Read the model definition and answer for the solid it produces. Units are mm, in the model's axes. Face numbers are marked on the shaded views. A direction names the side the tool comes from. Round coordinates to 2 decimals unless told otherwise and drop trailing zeros. Write each loop counter-clockwise with the first axis right and the second up, starting at its lowest first coordinate (ties: lowest second). Pieces come first, ordered by that corner, then holes. Notation, with made-up numbers: (-20, -9) -> (-3, -9) arc R6 cw to (-3, 1) -> close; hole circle Ø2 at (13, 86). An arc over 180 degrees is marked (long way). Return JSON: item names as keys, results as strings.
from build123d import *

# Parameters (mm, degrees)
SKETCH1_R                  = 1.75
BOSS_EXTRUDE1_DEPTH        = 1
BOSS_EXTRUDE2_START        = -1
BOSS_EXTRUDE2_DEPTH        = 1
SKETCHED_START             = 7.177417197
SKETCHED_BEND1_OUTLINE_R   = 1.75
SKETCHED_BEND1_DEPTH       = 1.366025404
SKETCHED_START_2           = -14
SKETCHED_BEND1_2_DEPTH     = 14
SKETCHED_START_3           = -6
SKETCHED_BEND1_3_DEPTH     = 5
SKETCHED_START_4           = -1.253227831
SKETCHED_BEND1_4_DEPTH     = 1.253227831
SKETCHED_START_5           = -6.500618506
SKETCHED_BEND1_5_DEPTH     = 0.500618506
SKETCHED_START_6           = -0.400872669
SKETCHED_BEND1_6_OUTLINE_R = 1.75
SKETCHED_BEND1_6_DEPTH     = 1


with BuildPart() as part:
    # Sketch1 → Boss-Extrude1 (new body)
    with BuildSketch(Plane(origin=(0, 0, 0), x_dir=(1, 0, 0), z_dir=(0, 1, 0))):
        with BuildLine():
            Line((-9.134882229, 6), (2.865117771, 6))
            Line((2.865117771, 6), (2.865117771, 8.250618606))
            ThreePointArc((2.865117771, 8.250618606), (6.365117771, 11.750618606), (9.865117771, 8.250618606))
            Line((9.865117771, 8.250618606), (9.865117771, 6))
            Line((9.865117771, 6), (9.865117771, 1))
            ThreePointArc((9.865117771, 1), (9.572224552, 0.292893219), (8.865117771, 0))
            Line((8.865117771, 0), (-9.134882229, 0))
            ThreePointArc((-9.134882229, 0), (-9.84198901, 0.292893219), (-10.134882229, 1))
            Line((-10.134882229, 1), (-10.134882229, 5))
            ThreePointArc((-10.134882229, 5), (-9.84198901, 5.707106781), (-9.134882229, 6))
        make_face()
        with Locations(Location((6.365117771, 8.250618606, 0), (0, 0, 270))):
            Circle(SKETCH1_R, mode=Mode.SUBTRACT)
    extrude(amount=BOSS_EXTRUDE1_DEPTH)

    # Sketch3 → Boss-Extrude2 (add)
    with BuildSketch(Plane(origin=(0, 1, 0), x_dir=(1, 0, 0), z_dir=(0, 1, 0)).offset(BOSS_EXTRUDE2_START)):
        with BuildLine():
            Line((8.17494801, 12.885336532), (7.42494801, 11.586298426))
            ThreePointArc((7.42494801, 11.586298426), (8.115117771, 11.281707519), (8.723986115, 10.836298426))
            Line((8.723986115, 10.836298426), (9.473986115, 12.135336532))
            Line((9.473986115, 12.135336532), (8.17494801, 12.885336532))
        make_face()
    extrude(amount=BOSS_EXTRUDE2_DEPTH)

    # Sketched Bend1: read off the stored shape, not the designer's step
    # Sketched Bend1 outline → Sketched Bend1 (cut)
    with BuildSketch(Plane(origin=(0, 0, 0), x_dir=(0.49999999999999767, 0.86602540378444, 0), z_dir=(0.8660254037844399, -0.49999999999999795, 0)).offset(SKETCHED_START)):
        with Locations((7.402836748, -8.250618606)):
            Circle(SKETCHED_BEND1_OUTLINE_R)
    extrude(amount=SKETCHED_BEND1_DEPTH, mode=Mode.SUBTRACT)

    # Sketched Bend1 2 outline → Sketched Bend1 2 (cut)
    with BuildSketch(Plane.XY.offset(SKETCHED_START_2)):
        with BuildLine():
            Line((-0.626369748, 1), (-1.955441123, 0.232660284))
            ThreePointArc((-1.955441123, 0.232660284), (-2.374275969, 0.05917321), (-2.823741123, 0))
            Line((-2.823741123, 0), (9.865117771, 0))
            Line((9.865117771, 0), (9.865117771, 1))
            Line((9.865117771, 1), (-0.626369748, 1))
        make_face()
    extrude(amount=SKETCHED_BEND1_2_DEPTH, mode=Mode.SUBTRACT)

    # Sketched Bend1 3 outline → Sketched Bend1 3 (add)
    with BuildSketch(Plane.XY.offset(SKETCHED_START_3)):
        with BuildLine():
            ThreePointArc((1.583564135, 3.544558877), (1.466504678, 3.392004022), (1.313949823, 3.274944565))
            Line((1.313949823, 3.274944565), (-2.455441123, 1.098685688))
            ThreePointArc((-2.455441123, 1.098685688), (-2.633095014, 1.025099036), (-2.823741123, 1))
            Line((-2.823741123, 1), (-0.626369748, 1))
            Line((-0.626369748, 1), (1.813949823, 2.408919161))
            ThreePointArc((1.813949823, 2.408919161), (2.173611459, 2.684897241), (2.449589539, 3.044558877))
            Line((2.449589539, 3.044558877), (5.970277863, 9.142569932))
            Line((5.970277863, 9.142569932), (5.104252459, 9.642569932))
            Line((5.104252459, 9.642569932), (1.583564135, 3.544558877))
        make_face()
    extrude(amount=SKETCHED_BEND1_3_DEPTH)

    # Sketched Bend1 4 outline → Sketched Bend1 4 (add)
    with BuildSketch(Plane.XY.offset(SKETCHED_START_4)):
        with BuildLine():
            ThreePointArc((1.583564135, 3.544558877), (1.466504678, 3.392004022), (1.313949823, 3.274944565))
            Line((1.313949823, 3.274944565), (-2.455441123, 1.098685688))
            ThreePointArc((-2.455441123, 1.098685688), (-2.633095014, 1.025099036), (-2.823741123, 1))
            Line((-2.823741123, 1), (-0.626369748, 1))
            Line((-0.626369748, 1), (1.813949823, 2.408919161))
            ThreePointArc((1.813949823, 2.408919161), (2.173611459, 2.684897241), (2.449589539, 3.044558877))
            Line((2.449589539, 3.044558877), (2.470277863, 3.080392105))
            Line((2.470277863, 3.080392105), (1.604252459, 3.580392105))
            Line((1.604252459, 3.580392105), (1.583564135, 3.544558877))
        make_face()
    extrude(amount=SKETCHED_BEND1_4_DEPTH)

    # Sketched Bend1 5 outline → Sketched Bend1 5 (add)
    with BuildSketch(Plane.XY.offset(SKETCHED_START_5)):
        Polygon((5.104252459, 9.642569932), (1.604252459, 3.580392105), (2.470277863, 3.080392105), (5.970277863, 9.142569932), align=None)
    extrude(amount=SKETCHED_BEND1_5_DEPTH)

    # Sketched Bend1 6 outline → Sketched Bend1 6 (add)
    with BuildSketch(Plane(origin=(0, 0, 0), x_dir=(0.49999999999999767, 0.86602540378444, 0), z_dir=(0.8660254037844399, -0.49999999999999795, 0)).offset(SKETCHED_START_6)):
        with BuildLine():
            Line((3.8614601, 0), (3.8614601, -6))
            Line((3.8614601, -6), (3.902836748, -6))
            Line((3.902836748, -6), (3.902836748, -8.250618606))
            ThreePointArc((3.902836748, -8.250618606), (5.336367033, -11.075455401), (8.462666987, -11.586298426))
            Line((8.462666987, -11.586298426), (9.212666987, -12.885336532))
            Line((9.212666987, -12.885336532), (10.511705093, -12.135336532))
            Line((10.511705093, -12.135336532), (9.761705093, -10.836298426))
            ThreePointArc((9.761705093, -10.836298426), (10.604870415, -9.663764174), (10.902836748, -8.250618606))
            Line((10.902836748, -8.250618606), (10.902836748, -1))
            ThreePointArc((10.902836748, -1), (10.609943529, -0.292893219), (9.902836748, 0))
            Line((9.902836748, 0), (3.8614601, 0))
        make_face()
        with Locations((7.402836748, -8.250618606)):
            Circle(SKETCHED_BEND1_6_OUTLINE_R, mode=Mode.SUBTRACT)
    extrude(amount=SKETCHED_BEND1_6_DEPTH)


solid = part.part
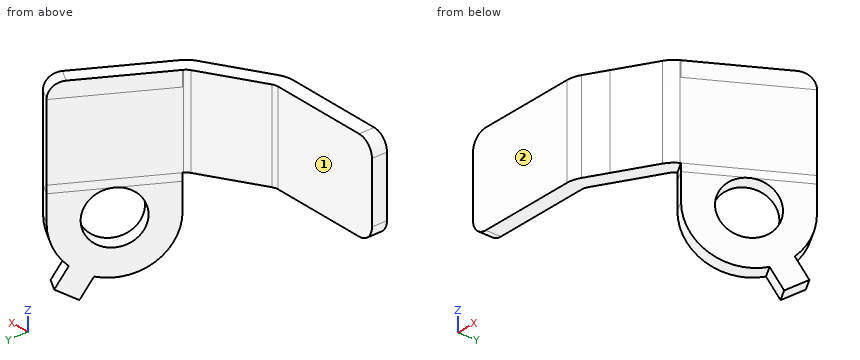
Item 1: Straight lines are drawn through the part: L1, parallel to X at y = 5.5, z = -11.25; L2, parallel to Y at x = 4.5, z = -12; L3, parallel to X at y = 8.5, z = -2.5. For each, find the intervals that lie inside material, in ascending order. Write a range as [from, to].
Worked answers:
{"L1": "x = [2.71, 3.87]", "L2": "y = [7.45, 8.6]", "L3": "x = [4.44, 5.6]"}
Item 2: Section A-A (z = -8.75) is taken. Give the vertices of the cut face in (x, y), then the cut area to 3 significant figures.
Worked answers:
{"outline": "(1.62, 3.61) -> (2.49, 3.11) -> (3.38, 4.66) -> (2.52, 5.16) -> close; (4.19, 8.06) -> (5.06, 7.56) -> (5.95, 9.11) -> (5.09, 9.61) -> close", "area": "3.57 mm2"}
Item 3: Flat-ended cylindrical pins translate along their axes: pin 1 (2 mm diameter, centred on y = 7, z = -10, fed in from +X); pin 2 (2 mm diameter, centred on x = 1.5, z = -11, fed in from +Y); pin 3 (3 mm diameter, centred on x = -3, y = 1, fed in from -Z). Find the tip coordinate at first contact, or state that the pin passes through.
Worked answers:
{"pin 1": "stops at x = 5.31", "pin 2": "stops at y = 5.13", "pin 3": "stops at z = -6"}
Item 4: Section C-C (z = -4.5) is taken. Give the vertices of the cut face in (x, y), then the cut area to 3 significant figures.
Worked answers:
{"outline": "(-10.13, 0) -> (-2.82, 0) arc R1.74 ccw to (-1.96, 0.23) -> (1.81, 2.41) arc R1.74 ccw to (2.45, 3.04) -> (5.97, 9.14) -> (5.1, 9.64) -> (1.58, 3.54) arc R0.74 cw to (1.31, 3.27) -> (-2.46, 1.1) arc R0.74 cw to (-2.82, 1) -> (-10.13, 1) -> close", "area": "20.0 mm2"}
Item 5: A tool of negligible diameter and unlimited length cuts with its end or side. For the marked faces 1 and 2, from which of +Z, -Z, +X, -X, +Y, -Y can it reach the whole face along a straight path? Write none if from no direction.
Worked answers:
{"face 1": "+Z, -Z, -X, +Y", "face 2": "+Z, -Z, +X, -X, -Y"}
Item 6: Section D-D (y = 1.75) is taken. Give the vertices of the cut face in (x, z), then the cut area to 3 significant figures.
Worked answers:
{"outline": "(-1.33, -6) -> (0.67, -6) -> (0.67, 0) -> (-1.33, 0) -> close", "area": "12.0 mm2"}
Item 7: Section B-B (x = -6) is taken. Give the vertices of the cut face in (y, z), then the cut area to 3 significant figures.
Worked answers:
{"outline": "(0, -6) -> (1, -6) -> (1, 0) -> (0, 0) -> close", "area": "6.00 mm2"}
